Build history of the part. All positions in model axes, mm. Round coordinates to 2 decimals unless told otherwise and drop trailing zeros. Order: outer loops, then holes, each group sorted by start corner. A loop starts at its lowest first (then second) coordinate and runs counter-clockwise, first axis right, second up. Notation, with made-up numbers: (-20.75, 10) -> (13.25, 10) arc R23 ccw to (13.25, 46) -> close; hole circle Ø7 at (-14.75, 25.25). An arc over 180 degrees is marked (long way). Write item = value, one per line.
from build123d import *

# Parameters (mm, degrees)
F1_DEPTH = 70
F4_DEPTH = 20
F6_DEPTH = 15
F7_W     = 5.162358
F7_H     = 3.251191
F8_DEPTH = 100


with BuildPart() as f1:
    # F0 (on Front) → F1 (new body)
    with BuildSketch(Plane.XZ):
        with BuildLine():
            Line((-0.5, 2.5), (-0.5, 1.936492))
            ThreePointArc((-0.5, 1.936492), (0, -2), (0.5, 1.936492))
            Line((0.5, 1.936492), (0.5, 2.5))
            Line((0.5, 2.5), (-0.5, 2.5))
        make_face()
    extrude(amount=F1_DEPTH)

    # F3 (on offset) → F4 (cut)
    with BuildSketch(Plane(origin=(0, -60, 0.089144), x_dir=(1, 0, 0), z_dir=(0, -1, 0))):
        with BuildLine():
            ThreePointArc((-0.5, 1.936492), (0.000638, 2), (0.501235, 1.936172))
            Line((0.501235, 1.936172), (0.5, 2.5))
            Line((0.5, 2.5), (-0.5, 2.5))
            Line((-0.5, 2.5), (-0.5, 1.936492))
        make_face()
    extrude(amount=-F4_DEPTH, mode=Mode.SUBTRACT)

    # F5 (on face) → F6 (cut)
    with BuildSketch(Plane.XZ.offset(60)):
        with BuildLine():
            Line((-0.5, 2.5), (-0.5, 1.936492))
            ThreePointArc((-0.5, 1.936492), (0, 2), (0.5, 1.936492))
            Line((0.5, 1.936492), (0.5, 2.5))
            Line((0.5, 2.5), (-0.5, 2.5))
        make_face()
    extrude(amount=-F6_DEPTH, mode=Mode.SUBTRACT)

    # F7 (on face) → F8 (cut)
    with BuildSketch(Plane.XZ.offset(70)):
        with Locations((0.0082, 1.625595)):
            Rectangle(F7_W, F7_H)
    extrude(amount=-F8_DEPTH, mode=Mode.SUBTRACT)


solid = f1.part
Q1. Probe probe 1 along X at (y, z) = (-67, -0.15); probe 2 along Z at (x, y) = (-0.55, -61); probe 3 along Z at (x, y) = (0.1, -12). List the from-to ranges inside material, lowest first.
Check values:
probe_1 = -1.99 to 1.99
probe_2 = -1.92 to 0
probe_3 = -2 to 0
Q2. Cut at A-A, the plane x = -1.2. List the corners of the cut face in (y, z), and give its area (3 significant figures).
Check values:
outline = (-70, -1.6) -> (0, -1.6) -> (0, 0) -> (-70, 0) -> close
area = 112 mm²
Q3. Flat gauge pin, fed straight in: pin 1 (1 mm diameter, centred on y = -8, z = -2, fed in from -X). Where does the tip first touch, or does it go through?
Check values:
pin_1 = -1.32
Q4. Cut at C-C, the plane z = -0.55. List the corners of the cut face in (x, y), and give its area (3 significant figures).
Check values:
outline = (-1.92, -70) -> (1.92, -70) -> (1.92, 0) -> (-1.92, 0) -> close
area = 269 mm²
Q5. Cut at B-B, the plane y = -41.5. List the corners of the cut face in (x, z).
Check values:
outline = (-2, 0) arc R2 ccw to (2, 0) -> close
Q6. Mould opens along X. For faces 1 (the face through (0, -35, 0)), 2 (the face through (0, -35, -2)) say: released by +X, released by -X, zero draft, split by the parting line, or undercut.
Check values:
face_1 = zero draft
face_2 = split by the parting line
